Input: dimensioned drawing with shaded views. Units: mm. Origin: part minimum x, y, z. Coordinates: 2 decimals unless noted, no trailing zeros. Write each loop counter-clockwise with the first axis right and the second up, starting at its lowest first coordinate (ties: lowest second). Pieces come first, ordered by that corner, then holes. Notation, with made-up numbers: M 44.25,12 L 50.25,12 A24 cw 50.25,34 Z; hole C -2.75,-19.75 d11. An arc over 180 degrees is marked long. Write each question's results on one line, items separated by ' | '. Start each with the question number.
1. Section query A-A, the plane x = 88.9. Output: boundary loops of the cut face in (y, z) (1 decimal), and give its area (3 significant figures).
2. Section query C-C, the plane z = 2.45. Output: boundary loops of the cut face in (x, y) (1 decimal), and give its area (3 significant figures).
3. Section query B-B, the plane y = 12.7. Output: boundary loops of the cut face in (x, z) (1 decimal).
4. Ray query, probe 1 along Y at (x, z) = (88.9, 0.85); probe 2 along X at (y, z) = (12.75, 1.65); probe 3 along Y at (x, z) = (25, 0.8) (1 decimal). Return the intervals inside material, ascending.
5. First-contact query: pin 1 (6 mm diameter, centred on x = 88.9, y = 12.7, fed in from -Z). Flat tip, straight axial feed; report the tip coordinate or a pass-through.
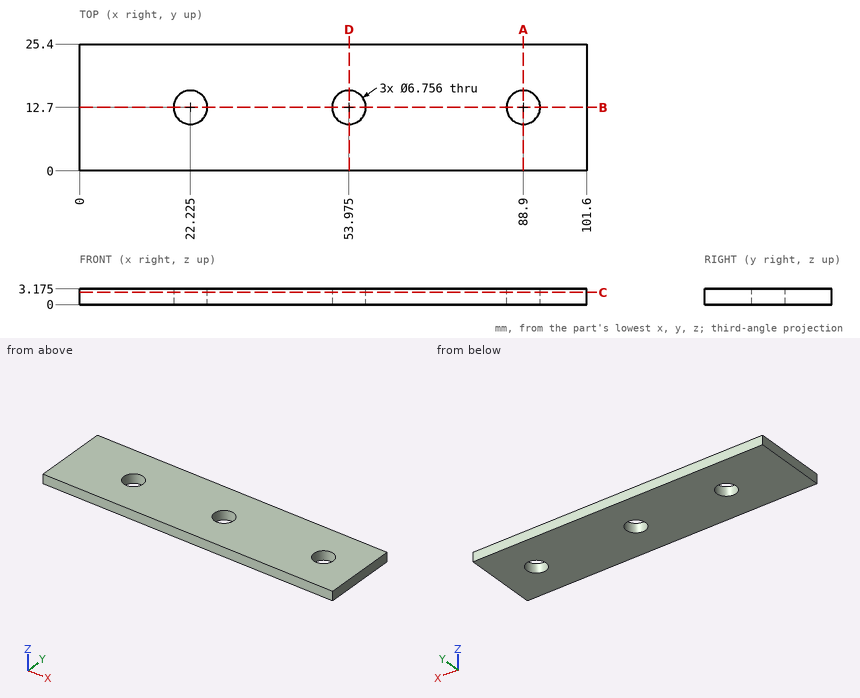
Answer:
1) outline: M 0,0 L 9.3,0 L 9.3,3.2 L 0,3.2 Z; M 16.1,0 L 25.4,0 L 25.4,3.2 L 16.1,3.2 Z | area: 59.2 mm^2
2) outline: M 0,0 L 101.6,0 L 101.6,25.4 L 0,25.4 Z; hole C 22.2,12.7 d6.8; hole C 54,12.7 d6.8; hole C 88.9,12.7 d6.8 | area: 2,470 mm^2
3) outline: M 0,0 L 18.8,0 L 18.8,3.2 L 0,3.2 Z; M 25.6,0 L 50.6,0 L 50.6,3.2 L 25.6,3.2 Z; M 57.4,0 L 85.5,0 L 85.5,3.2 L 57.4,3.2 Z; M 92.3,0 L 101.6,0 L 101.6,3.2 L 92.3,3.2 Z
4) probe 1: 0 to 9.32, 16.08 to 25.4 | probe 2: 0 to 18.85, 25.6 to 50.6, 57.35 to 85.52, 92.28 to 101.6 | probe 3: 0 to 10.8, 14.6 to 25.4
5) pin 1: through
